Part print with two shaded views. Sizes in mm from the minimum x, y, z corner. Give positions to 0.01 mm unless a question says otherwise; leave off trailing zeros. Write each loop counter-clockwise with the first axis right and the second up, starting at its lowest first coordinate (ties: lowest second). Pieces come first, ordered by that corner, then holes.
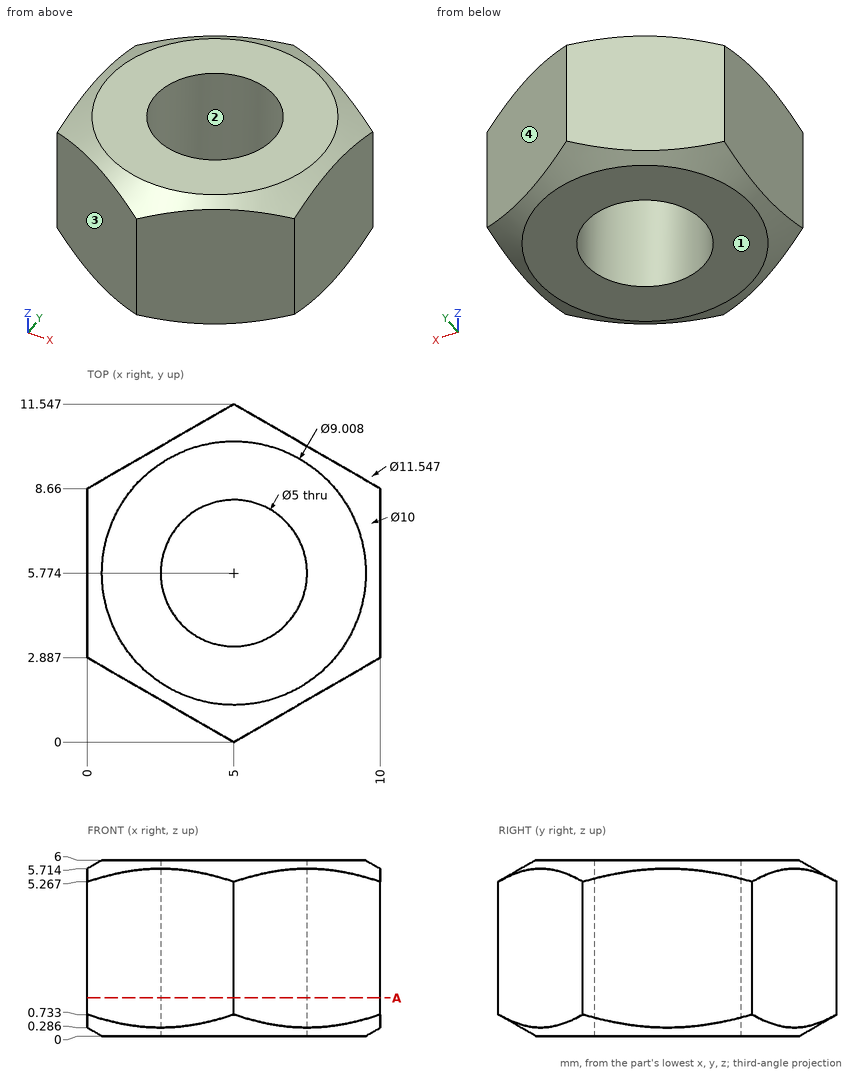
1) Mould opens along Y. For the marked faces 1, 2, 3 and 4 say: +Y half, -Y half, draft (parallel to the pull), parting line (faces both ways), or undercut.
Check result:
face 1: draft
face 2: undercut
face 3: -Y half
face 4: +Y half
2) Drill centre lines: L1, parallel to X at y = 4, z = 0.3 (1 decimal); L2, parallel to X at y = 5, z = 4.95; L3, parallel to Y at x = 3, z = 5.55 (1 decimal). Where is each one in solid material? Low to high.
Check result:
L1: x = 0.3 to 3.2, 6.8 to 9.7
L2: x = 0 to 2.62, 7.38 to 10
L3: y = 1.2 to 4.3, 7.3 to 10.4
3) Saw through at A-A (z = 1.3). Write the cut outline in (x, y).
Check result:
outline: (0, 2.89) - (5, 0) - (10, 2.89) - (10, 8.66) - (5, 11.55) - (0, 8.66) - close; hole circle Ø5 at (5, 5.77)
4) Flat gauge pins, fed straight in: P1, Ø2, axis at x = 3, z = 4.5, coming from the -Y side; P2, Ø2, axis at x = 4.5, z = 3.5, coming from the -Y side. Where does each tip first touch, or does it go through?
Check result:
P1: stops at y = 0.58
P2: stops at y = 0
